Geometry check sheet. Reference: the model listing, model coordinates, mm. Face numbers are marked on the shaded views. Coordinates: 2 decimals unless noted, no trailing zeros. One line per item, written item: value.
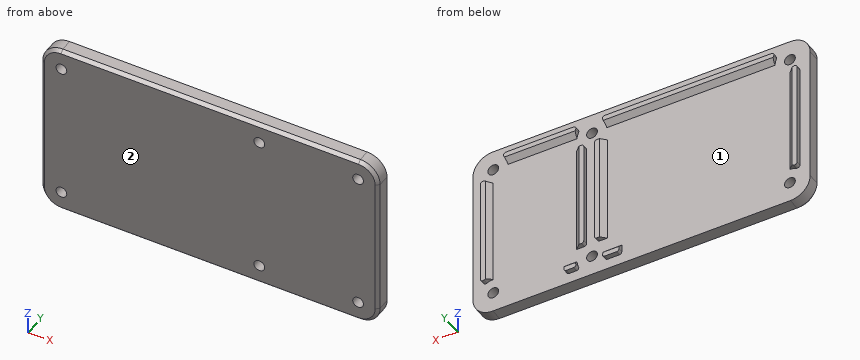
from build123d import *

# Parameters (mm, degrees)
BOSS_EXTRUDE1_DEPTH   = 4.7625
BOSS_EXTRUDE2_DEPTH   = 1.5875
SKETCH3_W             = 50.8
SKETCH3_H             = 1.5875
SKETCH3_W_2           = 20.32
CUT_EXTRUDE1_DEPTH    = 62.257755886
F_4_CLEARANCE_HOLE1_D = 3.4544
SKETCH6_R             = 4.7625
CUT_EXTRUDE2_DEPTH    = 62.257755886
SKETCH7_W             = 8.127020596
SKETCH7_H             = 2.415508094
SKETCH7_W_2           = 9.383301438
SKETCH7_H_2           = 3.436417543
CUT_EXTRUDE3_DEPTH    = 62.257755886
CHAMFER1_SIZE         = 1.5875
FILLET1_R             = 0.79375
CHAMFER2_SIZE         = 1.016


with BuildPart() as part:
    # Sketch1 → Boss-Extrude1 (new body)
    with BuildSketch(Plane(origin=(0, 0, 0), x_dir=(1, 0, 0), z_dir=(0, 1, 0))):
        with BuildLine():
            Line((-47.625, 28.575), (47.625, 28.575))
            ThreePointArc((47.625, 28.575), (52.115128061, 26.715128061), (53.975, 22.225))
            Line((53.975, 22.225), (53.975, -22.225))
            ThreePointArc((53.975, -22.225), (52.115128061, -26.715128061), (47.625, -28.575))
            Line((47.625, -28.575), (-47.625, -28.575))
            ThreePointArc((-47.625, -28.575), (-52.115128061, -26.715128061), (-53.975, -22.225))
            Line((-53.975, -22.225), (-53.975, 22.225))
            ThreePointArc((-53.975, 22.225), (-52.115128061, 26.715128061), (-47.625, 28.575))
        make_face()
    extrude(amount=BOSS_EXTRUDE1_DEPTH)

    # Sketch2 → Boss-Extrude2 (add)
    # profile 1 of 2: a face of its own
    with BuildSketch(Plane(origin=(0, 4.7625, 0), x_dir=(1, 0, 0), z_dir=(0, 1, 0))):
        with BuildLine():
            Line((-50.673, 22.225), (-50.673, -22.225))
            ThreePointArc((-50.673, -22.225), (-49.780261469, -24.380261469), (-47.625, -25.273))
            Line((-47.625, -25.273), (14.1605, -25.273))
            Line((14.1605, -25.273), (14.1605, 25.273))
            Line((14.1605, 25.273), (-47.625, 25.273))
            ThreePointArc((-47.625, 25.273), (-49.780261469, 24.380261469), (-50.673, 22.225))
        make_face()
        with BuildLine():
            Line((12.573, -23.6855), (-47.625, -23.6855))
            ThreePointArc((-47.625, -23.6855), (-48.657729454, -23.257729454), (-49.0855, -22.225))
            Line((-49.0855, -22.225), (-49.0855, 22.225))
            ThreePointArc((-49.0855, 22.225), (-48.657729454, 23.257729454), (-47.625, 23.6855))
            Line((-47.625, 23.6855), (12.573, 23.6855))
            Line((12.573, 23.6855), (12.573, -23.6855))
        make_face(mode=Mode.SUBTRACT)
    # profile 2 of 2: a face of its own
    with BuildSketch(Plane(origin=(0, 4.7625, 0), x_dir=(1, 0, 0), z_dir=(0, 1, 0))):
        with BuildLine():
            Line((47.625, -25.273), (17.5895, -25.273))
            Line((17.5895, -25.273), (17.5895, 25.273))
            Line((17.5895, 25.273), (47.625, 25.273))
            ThreePointArc((47.625, 25.273), (49.780261469, 24.380261469), (50.673, 22.225))
            Line((50.673, 22.225), (50.673, -22.225))
            ThreePointArc((50.673, -22.225), (49.780261469, -24.380261469), (47.625, -25.273))
        make_face()
        with BuildLine():
            Line((19.177, -23.6855), (19.177, 23.6855))
            Line((19.177, 23.6855), (47.625, 23.6855))
            ThreePointArc((47.625, 23.6855), (48.657729454, 23.257729454), (49.0855, 22.225))
            Line((49.0855, 22.225), (49.0855, -22.225))
            ThreePointArc((49.0855, -22.225), (48.657729454, -23.257729454), (47.625, -23.6855))
            Line((47.625, -23.6855), (19.177, -23.6855))
        make_face(mode=Mode.SUBTRACT)
    extrude(amount=BOSS_EXTRUDE2_DEPTH)

    # Sketch3 → Cut-Extrude1 (cut, through all)
    with BuildSketch(Plane(origin=(0, 4.7625, 0), x_dir=(1, 0, 0), z_dir=(0, 1, 0))):
        with Locations((-19.05, 24.47925)):
            Rectangle(SKETCH3_W, SKETCH3_H)
        with Locations((34.13125, 24.47925)):
            Rectangle(SKETCH3_W_2, SKETCH3_H)
    extrude(amount=CUT_EXTRUDE1_DEPTH, mode=Mode.SUBTRACT)

    # #4 Clearance Hole1 (through all)
    with Locations(Plane(origin=(0, 0, 0), x_dir=(-1, 0, 0), z_dir=(0, -1, 0))):
        with Locations((47.498, 22.098), (47.498, -22.098), (-15.875, -22.098), (-15.875, 22.098), (-47.498, 22.098), (-47.498, -22.098)):
            Hole(F_4_CLEARANCE_HOLE1_D / 2)

    # Sketch6 → Cut-Extrude2 (cut, through all)
    with BuildSketch(Plane(origin=(0, 4.7625, 0), x_dir=(1, 0, 0), z_dir=(0, 1, 0))):
        with Locations((47.498, 22.098)):
            Circle(SKETCH6_R)
        with Locations((47.498, -22.098)):
            Circle(SKETCH6_R)
        with Locations((15.875, -22.098)):
            Circle(SKETCH6_R)
        with Locations((15.875, 22.098)):
            Circle(SKETCH6_R)
        with Locations((-47.498, 22.098)):
            Circle(SKETCH6_R)
        with Locations((-47.498, -22.098)):
            Circle(SKETCH6_R)
    extrude(amount=CUT_EXTRUDE2_DEPTH, mode=Mode.SUBTRACT)

    # Sketch7 → Cut-Extrude3 (cut, through all)
    with BuildSketch(Plane(origin=(0, 4.7625, 0), x_dir=(1, 0, 0), z_dir=(0, 1, 0))):
        with Locations((15.913089186, 18.862568703)):
            Rectangle(SKETCH7_W, SKETCH7_H)
        with Locations((15.559399745, -19.373023428)):
            Rectangle(SKETCH7_W_2, SKETCH7_H_2)
    extrude(amount=CUT_EXTRUDE3_DEPTH, mode=Mode.SUBTRACT)

    # Chamfer1
    chamfer1_edges = [part.edges().sort_by_distance(p)[0] for p in [
        (-49.0855, 4.7625, 0),
        (8.86743597, 4.7625, -23.6855),
        (22.16818903, 4.7625, -23.6855),
        (49.0855, 4.7625, 0),
        (31.6865, 4.7625, 23.6855),
        (-15.8115, 4.7625, 23.6855),
        (12.573, 4.7625, 0),
        (19.177, 4.7625, 0),
    ]]
    chamfer(chamfer1_edges, length=CHAMFER1_SIZE - 0.0001)  # a hair under: the kernel refuses the full size

    # Fillet1
    fillet1_edges = [part.edges().sort_by_distance(p)[0] for p in [
        (6.35, 5.55625, -25.273),
        (23.97125, 5.55625, -25.273),
        (50.673, 5.55625, 18.548242086),
        (43.948242086, 5.55625, 25.273),
        (14.1605, 5.55625, 17.654814656),
        (17.5895, 5.55625, 17.654814656),
        (12.325242086, 5.55625, 25.273),
        (19.424757914, 5.55625, 25.273),
        (12.325242086, 5.55625, -25.273),
        (19.424757914, 5.55625, -25.273),
        (14.1605, 5.55625, -17.654814656),
        (17.5895, 5.55625, -17.654814656),
        (-50.673, 5.55625, -18.548242086),
        (-50.673, 5.55625, 18.548242086),
        (-43.948242086, 5.55625, 25.273),
        (50.673, 5.55625, -18.548242086),
    ]]
    fillet(fillet1_edges, radius=FILLET1_R)

    # Chamfer2
    chamfer2_edges = [part.edges().sort_by_distance(p)[0] for p in [
        (0, 0, -28.575),
        (52.115128061, 0, -26.715128061),
        (53.975, 0, 0),
        (52.115128061, 0, 26.715128061),
        (0, 0, 28.575),
        (-52.115128061, 0, 26.715128061),
        (-53.975, 0, 0),
        (-52.115128061, 0, -26.715128061),
    ]]
    chamfer(chamfer2_edges, length=CHAMFER2_SIZE)


solid = part.part
(1) Material ranges on probe 1 along X at (y, z) = (5.5, -11); probe 2 along X at (y, z) = (6, -3.5); probe 3 along Y at (x, z) = (-19, -6), recorded low to high. Write a range as from..to.
Reply:
probe 1: -50.67..-48.24, 11.72..14.16, 17.59..20.03, 48.24..50.67
probe 2: -50.67..-48.74, 12.22..14.16, 17.59..19.53, 48.74..50.67
probe 3: 0..4.76
(2) Release check for a two-part mould opening along X. For the marked faces 1 and 2 record: pulls with the +X half, pulls with the -X half, needs draft (parallel to the pull), parting line crosses it, or undercut.
Reply:
face 1: undercut
face 2: needs draft
(3) Go/stop test with flat-tipped pins: pin 1 Ø0.8 at (x, y) = (21.5, 6) entering from -Z; pin 2 Ø0.5 at (y, z) = (5.5, -0.5) entering from +X; pin 3 Ø0.8 at (y, z) = (5, -23.5) entering from -X; pin 4 Ø3 at (x, z) = (-47.498, -22.098) entering from -Y. Record where each tip stops, or that it passes through.
Reply:
pin 1: z = -25.27
pin 2: x = 50.67
pin 3: x = -53.9
pin 4: through
